from build123d import *

# Parameters (mm, degrees)
SKETCH1_W                 = 200
SKETCH1_H                 = 200
BOSS_EXTRUDE1_DEPTH       = 4
F_3_0MM_DOWEL_HOLE1_D     = 3
F_3_0MM_DOWEL_HOLE1_DEPTH = 4.001
MIRROR2_COPY_1_D          = 3
MIRROR2_COPY_1_DEPTH      = 4.001
CUT_EXTRUDE1_REACH        = 6
SKETCH6_R                 = 3


with BuildPart() as part:
    # Sketch1 → Boss-Extrude1 (new body)
    with BuildSketch(Plane.XY):
        Rectangle(SKETCH1_W, SKETCH1_H)
    extrude(amount=BOSS_EXTRUDE1_DEPTH)

    # Ø3.0mm Dowel Hole1
    with Locations(Plane.XY.offset(4)):
        with Locations((-80.25, 96.25), (-96.25, 96.25)):
            f_3_0mm_dowel_hole1 = Hole(F_3_0MM_DOWEL_HOLE1_D / 2, depth=F_3_0MM_DOWEL_HOLE1_DEPTH)

    # Mirror1: Ø3.0mm Dowel Hole1 across plane
    add(f_3_0mm_dowel_hole1.mirror(Plane.ZY), mode=Mode.SUBTRACT)

    # Mirror2: Ø3.0mm Dowel Hole1 across plane
    add(f_3_0mm_dowel_hole1.mirror(Plane.ZX), mode=Mode.SUBTRACT)

    # Mirror2 copy 1
    with Locations(Plane(origin=(0, 0, 4), x_dir=(-1, 0, 0), z_dir=(0, 0, 1))):
        with Locations((-80.25, 96.25), (-96.25, 96.25)):
            Hole(MIRROR2_COPY_1_D / 2, depth=MIRROR2_COPY_1_DEPTH)

    # Sketch6 → Cut-Extrude1 (cut, up to next)
    with BuildSketch(Plane(origin=(0, 0, 0), x_dir=(-1, 0, 0), z_dir=(0, 0, -1)), mode=Mode.PRIVATE) as cut_extrude1_sk1:
        with Locations((-40, 93)):
            Circle(SKETCH6_R)
    cut_extrude1_tool1 = extrude(cut_extrude1_sk1.sketch, amount=-CUT_EXTRUDE1_REACH, mode=Mode.PRIVATE) & part.part
    add(cut_extrude1_tool1.solids().sort_by_distance((40, 93, 0))[0], mode=Mode.SUBTRACT)
    # Sketch6 → Cut-Extrude1 (cut, up to next)
    with BuildSketch(Plane(origin=(0, 0, 0), x_dir=(-1, 0, 0), z_dir=(0, 0, -1)), mode=Mode.PRIVATE) as cut_extrude1_sk2:
        with Locations((40, 93)):
            Circle(SKETCH6_R)
    cut_extrude1_tool2 = extrude(cut_extrude1_sk2.sketch, amount=-CUT_EXTRUDE1_REACH, mode=Mode.PRIVATE) & part.part
    add(cut_extrude1_tool2.solids().sort_by_distance((-40, 93, 0))[0], mode=Mode.SUBTRACT)


solid = part.part
The model under review builds one solid part; all positions refer to its coordinate system, in mm. Give positions to 0.01 mm unless a question says otherwise; leave off trailing zeros. Write each loop counter-clockwise with the first axis right and the second up, starting at its lowest first coordinate (ties: lowest second). Pieces come first, ordered by that corner, then holes.
1. Add section A-A, the plane x = -40. Write out the cut boundary in (y, z), plus the area to 3 significant figures.
2. Wall thickness on L1, parallel to X at y = 96.25, z = 2.6; L2, parallel to Y at x = 96.25, z = 2.85: over which ranges is each line inside the solid? List them lowest first.
3. Draft analysis for pull direction Y (two halves, no side actions). For faces 1 (the cylindrical face through (-39.35, 90.07, 1.97)), 2 (the flat face through (-1, 1, 0)), state which applies: +Y half, -Y half, draft (parallel to the pull), parting line (faces both ways), or undercut.
Worked answers:
1. outline: (-100, 0) - (90, 0) - (90, 4) - (-100, 4) - close; (96, 0) - (100, 0) - (100, 4) - (96, 4) - close
1. area: 776 mm2
2. L1: x = -100 to -97.75, -94.75 to -81.75, -78.75 to 78.75, 81.75 to 94.75, 97.75 to 100
2. L2: y = -100 to -97.75, -94.75 to 94.75, 97.75 to 100
3. face 1: undercut
3. face 2: draft
